```python
from build123d import *
from OCP.BRepAlgoAPI import BRepAlgoAPI_Cut
from OCP.TopTools import TopTools_ListOfShape

# Parameters (mm, degrees)
SKETCH1_W            = 240
SKETCH1_H            = 140
BOSS_EXTRUDE2_DEPTH  = 20
DRAFT1_ANGLE         = 5.7
SKETCH4_W            = 90.996265389
SKETCH4_H            = 101.607418567
CUT_EXTRUDE1_DEPTH   = 2
CUT_EXTRUDE3_DEPTH   = 52
MIRROR2_COPY_1_DEPTH = 52
SKETCH6_R            = 57.5
SKETCH6_R_2          = 42
BOSS_EXTRUDE3_DEPTH  = 75
SKETCH7_W            = 6
SKETCH7_H            = 10
CUT_EXTRUDE4_DEPTH   = 10
SKETCH8_W            = 2
SKETCH8_H            = 45


with BuildPart() as part:
    # Sketch1 → Boss-Extrude2 (new body)
    with BuildSketch(Plane.XY):
        Rectangle(SKETCH1_W, SKETCH1_H)
    extrude(amount=BOSS_EXTRUDE2_DEPTH)

    # Draft1
    draft1_faces = [part.faces().sort_by_distance(p)[0] for p in [
        (120, 0, 10),
        (-120, 0, 10),
    ]]
    draft(draft1_faces, Plane.XY.offset(20), DRAFT1_ANGLE)

    # Sketch4 → Cut-Extrude1 (cut)
    with BuildSketch(Plane(origin=(0, 0, 0), x_dir=(-1, 0, 0), z_dir=(0, 0, -1))):
        with Locations((-57.498132695, -0.196290716)):
            Rectangle(SKETCH4_W, SKETCH4_H)
        with Locations((57.498132695, -0.196290716)):
            Rectangle(SKETCH4_W, SKETCH4_H)
    extrude(amount=-CUT_EXTRUDE1_DEPTH, mode=Mode.SUBTRACT)

    # Sketch5 → Cut-Extrude3 (cut)
    with BuildSketch(Plane(origin=(0, 0, 0), x_dir=(-1, 0, 0), z_dir=(0, 0, -1))):
        with BuildLine():
            Line((-92.996265389, 24), (-86.996265389, 24))
            ThreePointArc((-86.996265389, 24), (-78.996265389, 32), (-86.996265389, 40))
            Line((-86.996265389, 40), (-92.996265389, 40))
            ThreePointArc((-92.996265389, 40), (-100.996265389, 32), (-92.996265389, 24))
        make_face()
    cut_extrude3 = extrude(amount=-CUT_EXTRUDE3_DEPTH, mode=Mode.SUBTRACT)

    # Mirror1: Cut-Extrude3 across plane
    add(cut_extrude3.mirror(Plane(origin=(0, 0, 0), x_dir=(0, 0, 1), z_dir=(1, 0, 0))), mode=Mode.SUBTRACT)

    # Mirror2: Cut-Extrude3 across plane
    add(cut_extrude3.mirror(Plane.ZX), mode=Mode.SUBTRACT)

    # Mirror2 copy 1 sketch → Mirror2 copy 1 (cut)
    with BuildSketch(Plane(origin=(0, 0, 0), x_dir=(1, 0, 0), z_dir=(0, 0, -1))):
        with BuildLine():
            Line((-92.996265389, 24), (-86.996265389, 24))
            ThreePointArc((-86.996265389, 24), (-78.996265389, 32), (-86.996265389, 40))
            Line((-86.996265389, 40), (-92.996265389, 40))
            ThreePointArc((-92.996265389, 40), (-100.996265389, 32), (-92.996265389, 24))
        make_face()
    extrude(amount=-MIRROR2_COPY_1_DEPTH, mode=Mode.SUBTRACT)

    # Sketch6 → Boss-Extrude3 (add)
    with BuildSketch(Plane.XY.offset(20)):
        with Locations(Location((0, 0, 0), (0, 0, 180))):
            Circle(SKETCH6_R)
        Circle(SKETCH6_R_2, mode=Mode.SUBTRACT)
    extrude(amount=BOSS_EXTRUDE3_DEPTH)

    # Sketch7 → Cut-Extrude4 (cut)
    with BuildSketch(Plane.XY.offset(95)):
        with Locations((-42, 0)):
            Rectangle(SKETCH7_W, SKETCH7_H)
    extrude(amount=-CUT_EXTRUDE4_DEPTH, mode=Mode.SUBTRACT)


with BuildPart() as cut_revolve1_tool:
    # Sketch8 → Cut-Revolve1 (revolve)
    with BuildSketch(Plane(origin=(0, 0, 0), x_dir=(1, 0, 0), z_dir=(0, 1, 0))):
        with Locations((-43.000000734, -56.5)):
            Rectangle(SKETCH8_W, SKETCH8_H)
    revolve(axis=Axis((0, 0, 0), (0, 0, 1)))


with BuildPart() as part_1:
    add(part.part)

    # Cut-Revolve1: cut by cut_revolve1_tool, with a tolerance
    cut_revolve1_stock = TopTools_ListOfShape()
    cut_revolve1_stock.Append(part_1.part.wrapped)
    cut_revolve1_tools = TopTools_ListOfShape()
    cut_revolve1_tools.Append(cut_revolve1_tool.part.wrapped)
    cut_revolve1_cut = BRepAlgoAPI_Cut()
    cut_revolve1_cut.SetArguments(cut_revolve1_stock)
    cut_revolve1_cut.SetTools(cut_revolve1_tools)
    cut_revolve1_cut.SetFuzzyValue(0.00001)
    cut_revolve1_cut.Build()
    add(Compound.cast(cut_revolve1_cut.Shape()).solids(), mode=Mode.REPLACE)


solid = part_1.part
```
Geometry check sheet. Reference: the model listing, model coordinates, mm. A direction names the side the tool comes from. Round coordinates to 2 decimals unless told otherwise and drop trailing zeros. Order: outer loops, then holes, each group sorted by start corner. A loop starts at its lowest first (then second) coordinate and runs counter-clockwise, first axis right, second up. Notation, with made-up numbers: (-3.75, -11) - (53.25, -11) arc R29 cw to (53.25, 14) - close; hole circle Ø6 at (55, 20.25). An arc over 180 degrees is marked (long way). Use a Markdown table: item, result. Add a question column.
1) Gauge pin test, flat ends, axial feed: P1, Ø2, axis at y = 23, z = 1, coming from the +X side; P2, Ø0.6, axis at y = 9, z = 0.5, coming from the -X side; P3, Ø10, axis at y = -36, z = 54.5, coming from the +X side; P4, Ø1.5, axis at y = -39, z = 44.5, coming from the +X side. Record the tip position at first contact, or that the pin passes through.
2) Section check C-C (y = -32). Count the separate pieces of the cut face and the enclosed holes in it, then the cut area to 3 significant figures.
3) Set-up check for faces 4 (the cylindrical face through (79, 31.8, 10.9)), 5 (the flat face through (-39, 16, 79)), 6 (the flat face through (-57, 1, 2)), 7 (the cylindrical face through (40.06, 12.62, 86.89)): record each of +Z, -Z, +X, -X, +Y, -Y from which the full face is reachable in a straight line by a thin tool's end or side.
4) Section check A-A (x = 67). Record the cut outline in (y, z).
5) Thickness scan on line 1 along Y through (x, z) = (0, 83.25); line 2 along X through (y, z) = (2, 27.5); line 3 along Z through (x, y) = (-75.5, -1). Record the ranges inside material, lowest first.
6) Section check B-B (z = 57). Record the cut outline in (x, y).
7) Section check D-D (x = 0). Record the cut outline in (y, z).
8) Mould release check, pull along Y, two halves, no side actions. Record for faces 1 (the flat face through (52, 32, 20)), 2 (the flat face through (-2, 70, 10)), 3 (the cylindrical face through (100.994, -32.176, 10.874)): released by +Y, released by -Y, zero draft, split by the parting line, or undercut.
Established:
| question | item | result |
|---|---|---|
| 1 | P1 | x = 122 |
| 1 | P2 | x = -121.98 |
| 1 | P3 | x = 48.43 |
| 1 | P4 | x = 42.93 |
| 2 | separate pieces | 3 |
| 2 | enclosed holes | 0 |
| 2 | area | 6,500 mm2 |
| 3 | face 4 | +Z, -Z |
| 3 | face 5 | none |
| 3 | face 6 | -Z |
| 3 | face 7 | +Z |
| 4 | outline | (-70, 0) - (-51, 0) - (-51, 2) - (50.61, 2) - (50.61, 0) - (70, 0) - (70, 20) - (-70, 20) - close |
| 5 | line 1 | -57.5 to -42, 42 to 57.5 |
| 5 | line 2 | -57.47 to -41.95, 41.95 to 57.47 |
| 5 | line 3 | 2 to 20 |
| 6 | outline | circle Ø115 at (0, 0); hole circle Ø88 at (0, 0) |
| 7 | outline | (-70, 0) - (70, 0) - (70, 20) - (57.5, 20) - (57.5, 95) - (42, 95) - (42, 79) - (44, 79) - (44, 34) - (42, 34) - (42, 20) - (-42, 20) - (-42, 34) - (-44, 34) - (-44, 79) - (-42, 79) - (-42, 95) - (-57.5, 95) - (-57.5, 20) - (-70, 20) - close |
| 8 | face 1 | zero draft |
| 8 | face 2 | released by +Y |
| 8 | face 3 | undercut |
